Part model, mm, in its own coordinate system. A direction names the side the tool comes from. Give positions to 0.01 mm unless a question says otherwise; leave off trailing zeros. Order: outer loops, then holes, each group sorted by start corner. A loop starts at its lowest first (then second) coordinate and runs counter-clockwise, first axis right, second up. Notation, with made-up numbers: (-18.5, -29) - (-4.5, -29) arc R25 cw to (-4.5, 7) - close; hole circle Ø2 at (52.5, 4.25). An arc over 180 degrees is marked (long way). One line per item, written item: value.
```python
from build123d import *

# Parameters (mm, degrees)
ESQUISSE1_R             = 1
ESQUISSE1_RX            = 1
ESQUISSE1_RY            = 0.999955708
EXTRUSION1_DEPTH        = 9.3
EXTRUSION2_DEPTH        = 1
ENL_V_MAT_EXTRU_1_REACH = 53.345
ESQUISSE3_W             = 7.649288298
ESQUISSE3_H             = 26
ENL_V_MAT_EXTRU_2_REACH = 53.345
ESQUISSE4_W             = 6.951833508
ESQUISSE4_H             = 37
ENL_V_MAT_EXTRU_3_DEPTH = 9
CHANFREIN1_SIZE         = 5
ENL_V_MAT_EXTRU_4_DEPTH = 8


with BuildPart() as part:
    # Esquisse1 → Extrusion1 (new body)
    with BuildSketch(Plane.XY):
        with BuildLine():
            Line((22, 0), (22, 25))
            Line((22, 25), (0, 25))
            Line((0, 25), (0, -10))
            Line((0, -10), (22, -10))
            Line((22, -10), (22, -11))
            Line((22, -11), (21.190138404, -13.124684482))
            ThreePointArc((21.190138404, -13.124684482), (18.28157598, -15.158841298), (15.373013556, -13.124684482))
            Line((15.373013556, -13.124684482), (14.596979988, -11))
            Line((14.596979988, -11), (-1, -11))
            Line((-1, -11), (-1, 26))
            Line((-1, 26), (7.292692784, 26))
            Line((7.292692784, 26), (7.292692784, 41.355378005))
            Line((7.292692784, 41.355378005), (9.96388584, 44.427250018))
            Line((9.96388584, 44.427250018), (11.43304202, 44.427250018))
            Line((11.43304202, 44.427250018), (14.596979988, 41.355378005))
            Line((14.596979988, 41.355378005), (14.596979988, 26))
            Line((14.596979988, 26), (23, 26))
            Line((23, 26), (23, 0))
            Line((23, 0), (22, 0))
        make_face()
        with Locations((10.835624977, 29.282154136)):
            Circle(ESQUISSE1_R, mode=Mode.SUBTRACT)
        with Locations((10.835624977, 40.485887017)):
            Circle(ESQUISSE1_R, mode=Mode.SUBTRACT)
        with Locations(Location((18.28157598, -12.062342241), (0, 0, 0))):
            Ellipse(ESQUISSE1_RX, ESQUISSE1_RY, mode=Mode.SUBTRACT)
    extrude(amount=-EXTRUSION1_DEPTH)

    # Esquisse2 → Extrusion2 (add)
    with BuildSketch(Plane.XY):
        Polygon((22, 0), (23, 0), (23, 26), (-1, 26), (-1, -11), (22, -11), align=None)
    extrude(amount=EXTRUSION2_DEPTH)

    # Enlèv. mat.-Extru.1: up to this face of the body (flat: up to its plane)
    enl_v_mat_extru_1_end = Plane(part.part.faces().sort_by_distance((14.596979988, 33.677689002, -4.65))[0])
    # Esquisse3 → Enlèv. mat.-Extru.1 (cut, up to the picked face)
    with BuildSketch(Plane(origin=(23, 0, 0), x_dir=(0, 0, -1), z_dir=(1, 0, 0)), mode=Mode.PRIVATE) as enl_v_mat_extru_1_sk1:
        with Locations((5.475355851, 13)):
            Rectangle(ESQUISSE3_W, ESQUISSE3_H)
    enl_v_mat_extru_1_tool1 = split(extrude(enl_v_mat_extru_1_sk1.sketch, amount=-ENL_V_MAT_EXTRU_1_REACH, mode=Mode.PRIVATE), bisect_by=enl_v_mat_extru_1_end, keep=Keep.BOTH, mode=Mode.PRIVATE)
    add(enl_v_mat_extru_1_tool1.solids().sort_by(Axis((23, 13, -5.475356), (-1, 0, 0)))[0], mode=Mode.SUBTRACT)

    # Enlèv. mat.-Extru.2: up to this face of the body (flat: up to its plane)
    enl_v_mat_extru_2_end = Plane(part.part.faces().sort_by_distance((7.292692784, 33.677689002, -4.65))[0])
    # Esquisse4 → Enlèv. mat.-Extru.2 (cut, up to the picked face)
    with BuildSketch(Plane.ZY.offset(1), mode=Mode.PRIVATE) as enl_v_mat_extru_2_sk1:
        with Locations((-5.824083246, 7.5)):
            Rectangle(ESQUISSE4_W, ESQUISSE4_H)
    enl_v_mat_extru_2_tool1 = split(extrude(enl_v_mat_extru_2_sk1.sketch, amount=-ENL_V_MAT_EXTRU_2_REACH, mode=Mode.PRIVATE), bisect_by=enl_v_mat_extru_2_end, keep=Keep.BOTH, mode=Mode.PRIVATE)
    add(enl_v_mat_extru_2_tool1.solids().sort_by(Axis((-1, 7.5, -5.824083), (1, 0, 0)))[0], mode=Mode.SUBTRACT)

    # Esquisse5 → Enlèv. mat.-Extru.3 (cut)
    with BuildSketch(Plane.XY.offset(1)):
        Polygon((8.576662765, 24.450773838), (13.66977831, 24.450773838), (13.66977831, 26), (14.010433901, 26), (14.010433901, 32.678482304), (15.670246393, 32.678482304), (15.670246393, 45.814943355), (7.292692784, 45.814943355), (7.292692784, 32.678482304), (7.959479115, 32.678482304), (7.959479115, 26), (8.576662765, 26), align=None)
    extrude(amount=-ENL_V_MAT_EXTRU_3_DEPTH, mode=Mode.SUBTRACT)

    # Chanfrein1
    chanfrein1_edges = [part.edges().sort_by_distance(p)[0] for p in [
        (7.62608595, 32.678482304, 0),
        (14.303706945, 32.678482304, 0),
    ]]
    chamfer(chanfrein1_edges, length=CHANFREIN1_SIZE)

    # Esquisse6 → Enlèv. mat.-Extru.4 (cut)
    with BuildSketch(Plane.XY):
        with BuildLine():
            Line((22, -11), (14.596979988, -11))
            Line((14.596979988, -11), (15.373013556, -13.124684482))
            ThreePointArc((15.373013556, -13.124684482), (18.28157598, -15.158841298), (21.190138404, -13.124684482))
            Line((21.190138404, -13.124684482), (22, -11))
        make_face()
    extrude(amount=-ENL_V_MAT_EXTRU_4_DEPTH, mode=Mode.SUBTRACT)


solid = part.part
```
1) Two-plate mould, pull along Y, no slides. Class faces 1 (the face through (13, -11, -3)), 2 (the face through (14.01, 29, -5)), 3 (the face through (7.63, 30.14, -2.46)), 4 (the face through (13, -10, -5)): pulls with the +Y half, pulls with the -Y half, needs draft (parallel to the pull), parting line crosses it, or undercut.
Answer:
face 1: pulls with the -Y half
face 2: needs draft
face 3: pulls with the +Y half
face 4: undercut
2) Slice it at D-D on x = 1.75. Write the cut outline in (y, z).
Answer:
outline: (-11, -2.35) - (-10, -2.35) - (-10, 0) - (25, 0) - (25, -2.35) - (26, -2.35) - (26, 1) - (-11, 1) - close
3) Slice it at A-A on z = -7.25. Write the cut outline in (x, y).
Answer:
outline: (7.29, -11) - (22, -11) - (22, -10) - (7.29, -10) - close; (7.29, 25) - (8.58, 25) - (8.58, 26) - (7.96, 26) - (7.96, 32.68) - (7.29, 32.68) - close; (13.67, 25) - (14.6, 25) - (14.6, 32.68) - (14.01, 32.68) - (14.01, 26) - (13.67, 26) - close
4) Wall check: line 1 along Y through (x, z) = (8.5, -3); line 2 along Y through (x, z) = (14.75, -3.5); line 3 along Z through (x, y) = (21.25, -3.5). Give the ranges that are in metal, low to high. Write a range as [from, to].
Answer:
line 1: y = [-11, -10], [25, 26]
line 2: y = [-11, -10]
line 3: z = [0, 1]
5) Which spindle directions (+Z, -Z, +X, -X, +Y, -Y) get a long thin tool onto all of the face, cutting with end or side? Do faces 5 (the face through (15, -12.1, -8.6)), 6 (the face through (22.6, 15.8, -1.651)), 7 (the face through (7.959, 29, -5)), 8 (the face through (8, 25, -3)), 9 (the face through (11.1, 24.451, 0.5)). Say none if no direction does.
Answer:
face 5: +Z, -Z, -X, -Y
face 6: -Z, +X, +Y
face 7: +Z, +Y
face 8: -Z
face 9: +Z, -Z, +Y
6) Slice it at C-C on y = -8.5. Write the cut outline in (x, z).
Answer:
outline: (-1, -2.35) - (0, -2.35) - (0, 0) - (22, 0) - (22, 1) - (-1, 1) - close
7) Drop flat-ended pins along their axis: P1, Ø2, axis at y = 28, z = -3, coming from the -X side; P2, Ø2, axis at x = 2, z = -2, coming from the +Y side; P3, Ø2, axis at x = 12, y = 11.5, coming from the -Z side; P4, Ø1.2, axis at x = 10.84, y = 29.28, coming from the -Z side. Give the stop position or say it passes through.
Answer:
P1: stops at x = 7.29
P2: stops at y = 26
P3: stops at z = 0
P4: passes through
8) Slice it at B-B on x = 10.5. Write the cut outline in (y, z), then the cut area to 3 significant figures.
Answer:
outline: (-11, -9.3) - (-10, -9.3) - (-10, 0) - (24.45, 0) - (24.45, 1) - (-11, 1) - close; (25, -9.3) - (28.34, -9.3) - (28.34, -8) - (25, -8) - close; (30.22, -9.3) - (39.54, -9.3) - (39.54, -8) - (30.22, -8) - close; (41.43, -9.3) - (44.43, -9.3) - (44.43, -8) - (41.43, -8) - close
area: 65.1 mm2
